Part model, mm, in its own coordinate system. Face numbers are marked on the shaded views. Round coordinates to 2 decimals unless told otherwise and drop trailing zeros. Loops run counter-clockwise (first coordinate to the right, second up) from the corner with the lowest first, then second, coordinate; pieces in that order, holes last. Notation, with made-up numbers: (46.5, 85.5) - (102.5, 85.5) arc R20 ccw to (102.5, 120.5) - close; hole circle Ø4 at (-30, 7). An arc over 180 degrees is marked (long way). Put each result on its own line as item: value.
from build123d import *

# Parameters (mm, degrees)
F0_R     = 38.1
F0_R_2   = 31.75
F1_DEPTH = 123.825
F2_R     = 38.1
F3_DEPTH = 6.35
F4_R     = 5.08


with BuildPart() as f1:
    # F0 (on Front) → F1 (new body)
    with BuildSketch(Plane.XZ):
        Circle(F0_R)
        Circle(F0_R_2, mode=Mode.SUBTRACT)
    extrude(amount=F1_DEPTH)

    # F2 (on Front) → F3 (join)
    with BuildSketch(Plane.XZ):
        Circle(F2_R)
    extrude(amount=F3_DEPTH)

    # F4
    f4_edges = [f1.edges().sort_by_distance(p)[0] for p in [
        (-38.1, -123.825, 0),
    ]]
    fillet(f4_edges, radius=F4_R)


solid = f1.part
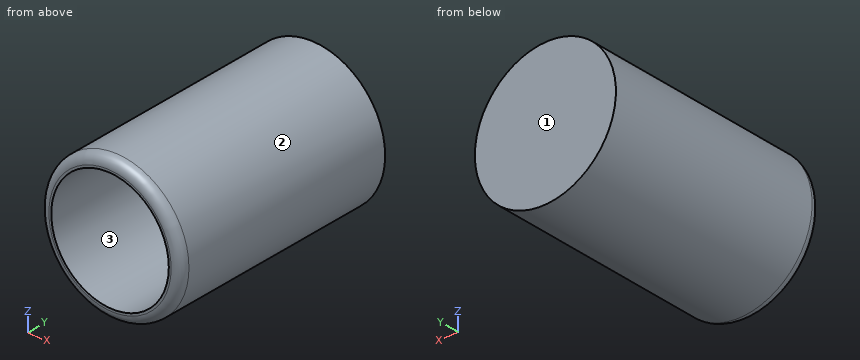
1. Band-saw the part on B-B (x = 0). List the corners of the cut face in (y, z) (3 decimals), plus the area to 3 significant figures.
A:
outline: (-123.825, -33.02) arc R5.08 ccw to (-118.745, -38.1) - (0, -38.1) - (0, 38.1) - (-118.745, 38.1) arc R5.08 ccw to (-123.825, 33.02) - (-123.825, 31.75) - (-6.35, 31.75) - (-6.35, -31.75) - (-123.825, -31.75) - close
area: 1,960 mm²
2. Probe line 1 along Z through (x, y) = (0, -85); line 2 along Y through (x, z) = (2.5, -11); line 3 along X through (y, z) = (-18, -27). List the from-to ranges inside material, lowest first. Write a range as [from, to].
A:
line 1: z = [-38.1, -31.75], [31.75, 38.1]
line 2: y = [-6.35, 0]
line 3: x = [-26.88, -16.71], [16.71, 26.88]
3. Pin check, flat tips, straight feed: P1, Ø12, axis at x = -16.5, y = -24.5, coming from the -Z side; P2, Ø5, axis at x = 16.5, y = -108.5, coming from the -Z side; P3, Ø5, axis at y = -23.5, z = -16.5, coming from the -X side. Stop position of each tip, or through.
A:
P1: stops at z = -36.62
P2: stops at z = -35.43
P3: stops at x = -35.43
4. Two-plate mould, pull along X, no slides. Class the marked faces 1, 2 and 3: pulls with the +X half, pulls with the -X half, needs draft (parallel to the pull), parting line crosses it, or undercut.
A:
face 1: needs draft
face 2: parting line crosses it
face 3: undercut
5. Band-saw the part on A-A (z = 0). List the corners of the cut face in (x, y) (3 decimals), plus the area to 3 significant figures.
A:
outline: (-38.1, -118.745) arc R5.08 ccw to (-33.02, -123.825) - (-31.75, -123.825) - (-31.75, -6.35) - (31.75, -6.35) - (31.75, -123.825) - (33.02, -123.825) arc R5.08 ccw to (38.1, -118.745) - (38.1, 0) - (-38.1, 0) - close
area: 1,960 mm²
6. Band-saw the part on C-C (y = -13). List the corners of the cut face in (x, z), plus the area to 3 significant figures.
A:
outline: circle Ø76.2 at (0, 0); hole circle Ø63.5 at (0, 0)
area: 1,390 mm²
